```python
from build123d import *

# Parameters (mm, degrees)
SKETCH_1_W                  = 120
SKETCH_1_H                  = 124
SKETCH_1_R                  = 39
EXTRUDE_1_DEPTH             = 6
SKETCH_2_R                  = 2.1
CUT_EXTRUDE_1_DEPTH         = 13
PATTERN_CIRCULAR_1_COUNT    = 8
SKETCH_3_R                  = 1.5
CUT_EXTRUDE_2_DEPTH         = 15
SKETCH_4_R                  = 1.5
CUT_EXTRUDE_5_DEPTH         = 10
HOLE_WIZARD_M5_1_AT_2_COUNT = 2
HOLE_WIZARD_M5_1_AT_2_PITCH = 45
HOLE_WIZARD_M5_1_AT_3_COUNT = 2
HOLE_WIZARD_M5_1_AT_3_PITCH = 90
HOLE_WIZARD_M5_2_AT_2_COUNT = 2
HOLE_WIZARD_M5_2_AT_2_PITCH = 45
HOLE_WIZARD_M5_2_AT_3_COUNT = 2
HOLE_WIZARD_M5_2_AT_3_PITCH = 90
SKETCH_10_W                 = 8
SKETCH_10_H                 = 10
CUT_EXTRUDE_6_DEPTH         = 13
HOLE_WIZARD_M5_3_D          = 4.2
CUT_EXTRUDE_7_DEPTH         = 13
PATTERN_CIRCULAR_2_COUNT    = 4
SKETCH_13_R                 = 5
CUT_EXTRUDE_8_DEPTH         = 13
PATTERN_CIRCULAR_3_COUNT    = 4
FILLET_1_R                  = 1


with BuildPart() as part:
    # 草图1 → 凸台-拉伸1 (new body, symmetric)
    with BuildSketch(Plane(origin=(0, 0, 0), x_dir=(1, 0, 0), z_dir=(0, 1, 0))):
        Rectangle(SKETCH_1_W, SKETCH_1_H)
        Circle(SKETCH_1_R, mode=Mode.SUBTRACT)
    extrude(amount=EXTRUDE_1_DEPTH, both=True)

    # 草图2 → 切除-拉伸1 (cut, through all)
    with BuildSketch(Plane(origin=(0, 6, 0), x_dir=(1, 0, 0), z_dir=(0, 1, 0))):
        with Locations((-16.072704159, 38.802940365)):
            Circle(SKETCH_2_R)
    cut_extrude_1 = extrude(amount=-CUT_EXTRUDE_1_DEPTH, mode=Mode.SUBTRACT)

    # 阵列(圆周)1: 切除-拉伸1 ×8 about axis
    pattern_circular_1_axis = Axis((0, 0, 0), (0, 1, 0))
    for i in range(1, PATTERN_CIRCULAR_1_COUNT):
        add(cut_extrude_1.rotate(pattern_circular_1_axis, i * 360 / PATTERN_CIRCULAR_1_COUNT), mode=Mode.SUBTRACT)

    # 草图3 → 切除-拉伸2 (cut)
    with BuildSketch(Plane(origin=(60, 0, 0), x_dir=(0, 0, -1), z_dir=(1, 0, 0))):
        with Locations((-45, 0)):
            Circle(SKETCH_3_R)
        Circle(SKETCH_3_R)
        with Locations((45, 0)):
            Circle(SKETCH_3_R)
    cut_extrude_2 = extrude(amount=-CUT_EXTRUDE_2_DEPTH, mode=Mode.SUBTRACT)

    # 草图4 → 切除-拉伸5 (cut)
    with BuildSketch(Plane(origin=(0, 0, -62), x_dir=(-1, 0, 0), z_dir=(0, 0, -1))):
        with Locations((-45, 0)):
            Circle(SKETCH_4_R)
        Circle(SKETCH_4_R)
        with Locations((45, 0)):
            Circle(SKETCH_4_R)
    cut_extrude_5 = extrude(amount=-CUT_EXTRUDE_5_DEPTH, mode=Mode.SUBTRACT)

    # 草图7 → M5 螺纹孔1 (revolve, cut)
    with BuildSketch(Plane(origin=(60, 0, -45), x_dir=(0, 0, -1), z_dir=(0, 1, 0))):
        Polygon((0, 0), (0, 18.6618073), (2.1, 17.4), (2.1, 0), align=None)
    hole_wizard_m5_1 = revolve(axis=Axis((66.35, 0, -45), (-1, 0, 0)), mode=Mode.SUBTRACT)

    # M5 螺纹孔1 at 2: M5 螺纹孔1 ×2
    with Locations(*[(0, 0, i * HOLE_WIZARD_M5_1_AT_2_PITCH) for i in range(1, HOLE_WIZARD_M5_1_AT_2_COUNT)]):
        add(hole_wizard_m5_1, mode=Mode.SUBTRACT)

    # M5 螺纹孔1 at 3: M5 螺纹孔1 ×2
    with Locations(*[(0, 0, i * HOLE_WIZARD_M5_1_AT_3_PITCH) for i in range(1, HOLE_WIZARD_M5_1_AT_3_COUNT)]):
        add(hole_wizard_m5_1, mode=Mode.SUBTRACT)

    # 草图9 → M5 螺纹孔2 (revolve, cut)
    with BuildSketch(Plane(origin=(45, 0, -62), x_dir=(0, 1, 0), z_dir=(1, 0, 0))):
        Polygon((0, 0), (0, 13.6618073), (2.1, 12.4), (2.1, 0), align=None)
    hole_wizard_m5_2 = revolve(axis=Axis((45, 0, -68.35), (0, 0, 1)), mode=Mode.SUBTRACT)

    # M5 螺纹孔2 at 2: M5 螺纹孔2 ×2
    with Locations(*[(-i * HOLE_WIZARD_M5_2_AT_2_PITCH, 0, 0) for i in range(1, HOLE_WIZARD_M5_2_AT_2_COUNT)]):
        add(hole_wizard_m5_2, mode=Mode.SUBTRACT)

    # M5 螺纹孔2 at 3: M5 螺纹孔2 ×2
    with Locations(*[(-i * HOLE_WIZARD_M5_2_AT_3_PITCH, 0, 0) for i in range(1, HOLE_WIZARD_M5_2_AT_3_COUNT)]):
        add(hole_wizard_m5_2, mode=Mode.SUBTRACT)

    # 镜向1: M5 螺纹孔1, 切除-拉伸2 across plane
    add(hole_wizard_m5_1.mirror(Plane(origin=(0, 0, 0), x_dir=(0, 0, 1), z_dir=(1, 0, 0))), mode=Mode.SUBTRACT)
    add(cut_extrude_2.mirror(Plane(origin=(0, 0, 0), x_dir=(0, 0, 1), z_dir=(1, 0, 0))), mode=Mode.SUBTRACT)

    # 镜向1 copy 1 sketch → 镜向1 copy 1 (revolve, cut)
    with BuildSketch(Plane(origin=(-60, 0, 0), x_dir=(0, 0, -1), z_dir=(0, 1, 0))):
        Polygon((0, 0), (0, -18.6618073), (2.1, -17.4), (2.1, 0), align=None)
    revolve(axis=Axis((-66.35, 0, 0), (-1, 0, 0)), mode=Mode.SUBTRACT)

    # 镜向1 copy 2 sketch → 镜向1 copy 2 (revolve, cut)
    with BuildSketch(Plane(origin=(-60, 0, 45), x_dir=(0, 0, -1), z_dir=(0, 1, 0))):
        Polygon((0, 0), (0, -18.6618073), (2.1, -17.4), (2.1, 0), align=None)
    revolve(axis=Axis((-66.35, 0, 45), (-1, 0, 0)), mode=Mode.SUBTRACT)

    # 镜向2: M5 螺纹孔2, 切除-拉伸5 across plane
    add(hole_wizard_m5_2.mirror(Plane.XY), mode=Mode.SUBTRACT)
    add(cut_extrude_5.mirror(Plane.XY), mode=Mode.SUBTRACT)

    # 镜向2 copy 1 sketch → 镜向2 copy 1 (revolve, cut)
    with BuildSketch(Plane(origin=(0, 0, 62), x_dir=(0, 1, 0), z_dir=(1, 0, 0))):
        Polygon((0, 0), (0, -13.6618073), (2.1, -12.4), (2.1, 0), align=None)
    revolve(axis=Axis((0, 0, 68.35), (0, 0, 1)), mode=Mode.SUBTRACT)

    # 镜向2 copy 2 sketch → 镜向2 copy 2 (revolve, cut)
    with BuildSketch(Plane(origin=(-45, 0, 62), x_dir=(0, 1, 0), z_dir=(1, 0, 0))):
        Polygon((0, 0), (0, -13.6618073), (2.1, -12.4), (2.1, 0), align=None)
    revolve(axis=Axis((-45, 0, 68.35), (0, 0, 1)), mode=Mode.SUBTRACT)

    # 草图10 → 切除-拉伸6 (cut, through all)
    with BuildSketch(Plane.XZ.offset(6)):
        with Locations((-56, 57)):
            Rectangle(SKETCH_10_W, SKETCH_10_H)
        with Locations((56, 57)):
            Rectangle(SKETCH_10_W, SKETCH_10_H)
        with Locations((56, -57)):
            Rectangle(SKETCH_10_W, SKETCH_10_H)
        with Locations((-56, -57)):
            Rectangle(SKETCH_10_W, SKETCH_10_H)
    extrude(amount=-CUT_EXTRUDE_6_DEPTH, mode=Mode.SUBTRACT)

    # M5 螺纹孔3 (through all)
    with Locations(Plane(origin=(16.072704159, 6, -38.802940365), x_dir=(0, 0, 1), z_dir=(0, 1, 0))):
        with Locations((0, 0), (22.730236206, 22.730236206), (54.875644524, 22.730236206), (77.60588073, 0), (77.60588073, -32.145408318), (54.875644524, -54.875644524), (22.730236206, -54.875644524), (0, -32.145408318)):
            Hole(HOLE_WIZARD_M5_3_D / 2)

    # 草图12 → 切除-拉伸7 (cut, through all)
    with BuildSketch(Plane.XZ.offset(6)):
        with BuildLine():
            Line((22.257359313, -41.656705713), (41.656705713, -22.257359313))
            ThreePointArc((41.656705713, -22.257359313), (50.141987088, -22.257359313), (50.141987088, -30.742640687))
            Line((50.141987088, -30.742640687), (30.742640687, -50.141987088))
            ThreePointArc((30.742640687, -50.141987088), (22.257359313, -50.141987088), (22.257359313, -41.656705713))
        make_face()
    cut_extrude_7 = extrude(amount=-CUT_EXTRUDE_7_DEPTH, mode=Mode.SUBTRACT)

    # 阵列(圆周)2: 切除-拉伸7 ×4 about axis
    pattern_circular_2_axis = Axis((0, 0, 0), (0, 1, 0))
    for i in range(1, PATTERN_CIRCULAR_2_COUNT):
        add(cut_extrude_7.rotate(pattern_circular_2_axis, i * 360 / PATTERN_CIRCULAR_2_COUNT), mode=Mode.SUBTRACT)

    # 草图13 → 切除-拉伸8 (cut, through all)
    with BuildSketch(Plane.XZ.offset(6)):
        with Locations((11.904178767, 53.696280392)):
            Circle(SKETCH_13_R)
        with Locations((-11.904178767, 53.696280392)):
            Circle(SKETCH_13_R)
    cut_extrude_8 = extrude(amount=-CUT_EXTRUDE_8_DEPTH, mode=Mode.SUBTRACT)

    # 阵列(圆周)3: 切除-拉伸8 ×4 about axis
    pattern_circular_3_axis = Axis((0, 0, 0), (0, 1, 0))
    for i in range(1, PATTERN_CIRCULAR_3_COUNT):
        add(cut_extrude_8.rotate(pattern_circular_3_axis, i * 360 / PATTERN_CIRCULAR_3_COUNT), mode=Mode.SUBTRACT)

    # 圆角1
    fillet_1_edges = [part.edges().sort_by_distance(p)[0] for p in [
        (-60, 0, -52),
        (-52, 0, -52),
        (-52, 0, -62),
        (60, 0, -52),
        (52, 0, -62),
        (52, 0, -52),
        (60, 0, 52),
        (52, 0, 52),
        (52, 0, 62),
        (-60, 0, 52),
        (-52, 0, 62),
        (-52, 0, 52),
    ]]
    fillet(fillet_1_edges, radius=FILLET_1_R)


solid = part.part
```
Work out the finished part from the listing and answer in its coordinate system (mm). A direction names the side the tool comes from. Give positions to 0.01 mm unless a question says otherwise; leave off trailing zeros. Order: outer loops, then holes, each group sorted by start corner. A loop starts at its lowest first (then second) coordinate and runs counter-clockwise, first axis right, second up. Notation, with made-up numbers: (61.25, 81) -> (94.25, 81) arc R10 ccw to (94.25, 96) -> close; hole circle Ø3 at (-6.75, 56.25). An arc over 180 degrees is marked (long way). Answer as CSV lines item,"result". Start each with the question number.
(1) Consider line 1 along Y through (x, z) = (48.25, 45); line 2 along X through (y, z) = (4, 22.5); line 3 along X through (y, z) = (2.5, -10). Determine where each line is inside the solid, lowest interval first.
(2) Which of the six approach directions +Z, -Z, +X, -X, +Y, -Y give full straight-line access (tool end or side, diameter ignored) to faces 4 (the flat face through (52, 0, -57)), 5 (the flat face through (40.578, -0.084, -40.307)), 6 (the cylindrical face through (-51.42, 0.8, -46.94))?
(3) Section A-A, the plane x = -10 is taken. Write down the section's boundary in (y, z), plus the area to 3 significant figures.
(4) Each of these flat-tipped pins is pushed along its axis until it touches: pin 1 Ø2.5 at (x, y) = (-45, 0) entering from -Z; pin 2 Ø2.5 at (y, z) = (1, 58) entering from +X; pin 3 Ø4 at (y, z) = (0, 0) entering from +X. Where does it stop, or does it pass through?
(5) Section B-B, the plane z = 35 is taken. Write down the section's boundary in (x, y).
(6) Section D-D, the plane y = 3.75 is taken. Give the number of separate pieces and of enclosed holes in the cut face, plus the area to 3 significant figures.
(7) For a pull along Y with two mould halves and no side action, classify faces 1 (the cylindrical face through (51.42, 0.8, 43.06)), 2 (the cylindrical face through (48.815, -0.084, 12.988)), 3 (the conical face through (44.69, 0.2, -48.56)) as released by +Y, released by -Y, zero draft, split by the parting line, or undercut.
(8) Section C-C, the plane z = 4 is taken. Write down the section's boundary in (x, y).
Entries:
1,line 1,"-6 to -2.1, 2.1 to 6"
1,line 2,"-60 to -50.37, -41.41 to -31.86, 31.86 to 41.41, 50.37 to 60"
1,line 3,"-60 to -58.32, -49.07 to -37.7, 37.7 to 49.07, 58.32 to 60"
2,face 4,"-Z, +X, +Y, -Y"
2,face 5,"+Y, -Y"
2,face 6,"-X"
3,outline,"(-6, -62) -> (6, -62) -> (6, -58.32) -> (-6, -58.32) -> close; (-6, -49.07) -> (6, -49.07) -> (6, -37.7) -> (-6, -37.7) -> close; (-6, 37.7) -> (6, 37.7) -> (6, 49.07) -> (-6, 49.07) -> close; (-6, 58.32) -> (6, 58.32) -> (6, 62) -> (-6, 62) -> close"
3,area,"361 mm²"
4,pin 1,"z = -49.09"
4,pin 2,"x = 52"
4,pin 3,"x = 42.54"
5,outline,"(-60, -6) -> (-45.88, -6) -> (-45.88, 6) -> (-60, 6) -> close; (-28.91, -6) -> (-17.2, -6) -> (-17.2, 6) -> (-28.91, 6) -> close; (17.2, -6) -> (28.91, -6) -> (28.91, 6) -> (17.2, 6) -> close; (45.88, -6) -> (60, -6) -> (60, 6) -> (45.88, 6) -> close"
6,separate pieces,"1"
6,enclosed holes,"21"
6,area,"7,270 mm²"
7,face 1,"undercut"
7,face 2,"zero draft"
7,face 3,"undercut"
8,outline,"(-60, -6) -> (-38.79, -6) -> (-38.79, 6) -> (-60, 6) -> close; (38.79, -6) -> (60, -6) -> (60, 6) -> (38.79, 6) -> close"
